Solid Edge part; units mm, degrees
sketch "Sketch1" plane through (0, 0, 0) normal (0, 0, 1) x (1, 0, 0)
  line L0 (-25, -25) -> (25, -25)
  line L1 (25, -25) -> (25, 25)
  line L2 (25, 25) -> (-25, 25)
  line L3 (-25, 25) -> (-25, -25)
  line L4 (-16.4, -17) -> (16.4, -17)
  line L5 (16.4, -17) -> (16.4, 17)
  line L6 (16.4, 17) -> (-16.4, 17)
  line L7 (-16.4, 17) -> (-16.4, -17)
  circle A0 centre (-20, -20) radius 1.7
  circle A1 centre (-20, 20) radius 1.7
  circle A2 centre (20, -20) radius 1.7
  circle A3 centre (20, 20) radius 1.7
extrude "Protrusion1" add sketch "Sketch1" along normal blind 4
Here's how the part is built. I have some questions about the finished solid (model axes, mm). A direction names the side the tool comes from. Round coordinates to 2 decimals unless told otherwise and drop trailing zeros. Loops run counter-clockwise (first coordinate to the right, second up) from the corner with the lowest first, then second, coordinate; pieces in that order, holes last.
1. If we section it at B-B on y = 7.5: Write out the boundary of the cut face in (x, z).
Answer list:
outline: (-25, 0) - (-16.4, 0) - (-16.4, 4) - (-25, 4) - close; (16.4, 0) - (25, 0) - (25, 4) - (16.4, 4) - close
2. For P1, Ø10, axis at x = 11.5, y = -11.5, coming from the +Z side, with a flat end and sliding along its axis, tell me the tip position at first contact or that it passes through.
Answer list:
P1: stops at z = 4
3. If we section it at D-D on z = 1.8: Write out the boundary of the cut face in (x, y), plus the area to 3 significant figures.
Answer list:
outline: (-25, -25) - (25, -25) - (25, 25) - (-25, 25) - close; hole circle Ø3.4 at (-20, -20); hole circle Ø3.4 at (-20, 20); hole (-16.4, -17) - (16.4, -17) - (16.4, 17) - (-16.4, 17) - close; hole circle Ø3.4 at (20, -20); hole circle Ø3.4 at (20, 20)
area: 1,350 mm2
4. If we section it at C-C on x = 20: Write out the boundary of the cut face in (y, z), plus the area to 3 significant figures.
Answer list:
outline: (-25, 0) - (-21.7, 0) - (-21.7, 4) - (-25, 4) - close; (-18.3, 0) - (18.3, 0) - (18.3, 4) - (-18.3, 4) - close; (21.7, 0) - (25, 0) - (25, 4) - (21.7, 4) - close
area: 173 mm2
5. If we section it at A-A on x = -3.5: Write out the boundary of the cut face in (y, z).
Answer list:
outline: (-25, 0) - (-17, 0) - (-17, 4) - (-25, 4) - close; (17, 0) - (25, 0) - (25, 4) - (17, 4) - close
6. We'd pull the mould along Y, two halves only. Please class faces 1 (the face through (21.57, -19.35, 1.97)), 2 (the face through (-17, 0, 0)), 3 (the face through (0, -25, 2)), 4 (the face through (-19.086, 18.567, 1.972)): +Y half, -Y half, draft (parallel to the pull), parting line (faces both ways), or undercut.
Answer list:
face 1: undercut
face 2: draft
face 3: -Y half
face 4: undercut
7. If I drill on line 1 along Y through (x, z) = (20, 2.9); line 2 along Y through (x, z) = (6, 1.8); line 3 along X through (y, z) = (10, 2.2), over which ranges is the centre line in solid material (lowest first)?
Answer list:
line 1: y = -25 to -21.7, -18.3 to 18.3, 21.7 to 25
line 2: y = -25 to -17, 17 to 25
line 3: x = -25 to -16.4, 16.4 to 25
8. Which directions (+Z, -Z, +X, -X, +Y, -Y) give clear straight access to the entire face, cutting with the end or side of a thin tool? Please do faces 5 (the face through (-16.4, 0, 2)), 6 (the face through (-25, 0, 2)).
Answer list:
face 5: +Z, -Z
face 6: +Z, -Z, -X, +Y, -Y
